Work out the finished part from the listing and answer in its coordinate system (mm). A direction names the side the tool comes from. Coordinates: 2 decimals unless noted, no trailing zeros. Loops run counter-clockwise (first coordinate to the right, second up) from the corner with the lowest first, then second, coordinate; pieces in that order, holes last. Notation, with made-up numbers: (81, -13) -> (131, -13) arc R14 cw to (131, 3) -> close; hole circle Ø7 at (-13.75, -25.5). An arc over 180 degrees is marked (long way). Use a Markdown table: item, result.
from build123d import *

# Parameters (mm, degrees)
F0_W     = 12.7
F0_H     = 11.2014
F3_DEPTH = 330.2


with BuildPart() as f1:
    # F0 (on Front) → F1 (revolve)
    with BuildSketch(Plane.XZ):
        Polygon((-228.391013, 31.75), (101.808987, 31.75), (101.808987, 50.8), (79.929347, 50.8), (-13.110853, 50.8), (-228.391013, 50.8), align=None)
        Polygon((-13.110853, 50.8), (79.929347, 50.8), (79.929347, 64.9986), (67.229347, 64.9986), (-13.110853, 64.9986), align=None)
        with Locations((73.579347, 70.5993)):
            Rectangle(F0_W, F0_H)
    revolve(axis=Axis((-0.204857, 0, 0), (-1, 0, 0)))

    # F2 (on face) → F3 (cut)
    with BuildSketch(Plane.YZ.offset(101.808987)):
        with BuildLine():
            Line((7.9375, 30.741805), (7.9375, 39.6875))
            Line((7.9375, 39.6875), (-7.9375, 39.6875))
            Line((-7.9375, 39.6875), (-7.9375, 30.741805))
            ThreePointArc((-7.9375, 30.741805), (0, 31.75), (7.9375, 30.741805))
        make_face()
    extrude(amount=-F3_DEPTH, mode=Mode.SUBTRACT)


solid = f1.part
Q1. Section C-C on x = 38 is taken. Determine the outline of the cut face in (y, z).
Solved:
| item | result |
|---|---|
| outline | circle Ø130 at (0, 0); hole (-7.94, 30.74) arc R31.75 ccw (long way) to (7.94, 30.74) -> (7.94, 39.69) -> (-7.94, 39.69) -> close |
Q2. For faces 4 (the flat face through (101.809, 23.3, -21.9)), 5 (the cylindrical face through (-122.258, -49.592, -11.012)), 6 (the flat face through (-61, -7.938, 35)), determine the directions among +Z, -Z, +X, -X, +Y, -Y from which every point of the face is accessible in a straight line to the end or side of a thin tool.
Solved:
| item | result |
|---|---|
| face 4 | +Z, -Z, +X, +Y, -Y |
| face 5 | -X |
| face 6 | +X, -X |
Q3. Determine the mould class of faces 1 (the flat face through (-61, 7.938, 35)), 2 (the flat face through (79.929, -16, -50)), 3 (the cylindrical face through (90.716, -49.592, -11.012)) for opening direction Y: pulls with the +Y half, pulls with the -Y half, needs draft (parallel to the pull), parting line crosses it, or undercut.
Solved:
| item | result |
|---|---|
| face 1 | undercut |
| face 2 | needs draft |
| face 3 | parting line crosses it |
Q4. Consider line 1 (Y direction, x = -14, z = 0); line 2 (Y direction, x = 5.5, z = 1.5); line 3 (Z direction, x = 37, y = -2). Determine where each line is inside the solid, lowest interval first. Write a range as [from, to].
Solved:
| item | result |
|---|---|
| line 1 | [-50.8, -31.75], [31.75, 50.8] |
| line 2 | [-64.98, -31.71], [31.71, 64.98] |
| line 3 | [-64.97, -31.69], [39.69, 64.97] |
Q5. Section D-D on y = -40 is taken. Determine the outline of the cut face in (x, z), and give its area (3 significant figures).
Solved:
| item | result |
|---|---|
| outline | (-228.39, -31.32) -> (-13.11, -31.32) -> (-13.11, -51.23) -> (67.23, -51.23) -> (67.23, -64.86) -> (79.93, -64.86) -> (79.93, -31.32) -> (101.81, -31.32) -> (101.81, 31.32) -> (79.93, 31.32) -> (79.93, 64.86) -> (67.23, 64.86) -> (67.23, 51.23) -> (-13.11, 51.23) -> (-13.11, 31.32) -> (-228.39, 31.32) -> close |
| area | 24,700 mm² |
Q6. Section A-A on z = 0 is taken. Determine the outline of the cut face in (x, y).
Solved:
| item | result |
|---|---|
| outline | (-228.39, -50.8) -> (-13.11, -50.8) -> (-13.11, -65) -> (67.23, -65) -> (67.23, -76.2) -> (79.93, -76.2) -> (79.93, -50.8) -> (101.81, -50.8) -> (101.81, -31.75) -> (-228.39, -31.75) -> close; (-228.39, 31.75) -> (101.81, 31.75) -> (101.81, 50.8) -> (79.93, 50.8) -> (79.93, 76.2) -> (67.23, 76.2) -> (67.23, 65) -> (-13.11, 65) -> (-13.11, 50.8) -> (-228.39, 50.8) -> close |
Q7. Section B-B on y = 0 is taken. Determine the outline of the cut face in (x, z).
Solved:
| item | result |
|---|---|
| outline | (-228.39, -50.8) -> (-13.11, -50.8) -> (-13.11, -65) -> (67.23, -65) -> (67.23, -76.2) -> (79.93, -76.2) -> (79.93, -50.8) -> (101.81, -50.8) -> (101.81, -31.75) -> (-228.39, -31.75) -> close; (-228.39, 39.69) -> (101.81, 39.69) -> (101.81, 50.8) -> (79.93, 50.8) -> (79.93, 76.2) -> (67.23, 76.2) -> (67.23, 65) -> (-13.11, 65) -> (-13.11, 50.8) -> (-228.39, 50.8) -> close |
Q8. Given pin 1 Ø5 at (x, y) = (-8.5, -17) entering from +Z; pin 2 Ø3 at (x, y) = (-58, 12.5) entering from +Z; pin 3 Ø10 at (x, z) = (17, 34) entering from -Y, each flat-ended and moving along its own axis, determine where each tip first touches the part or whether it passes through.
Solved:
| item | result |
|---|---|
| pin 1 | z = 63.36 |
| pin 2 | z = 49.59 |
| pin 3 | y = -58.17 |
